Work out the finished part from the listing and answer in its coordinate system (mm). A direction names the side the tool comes from. Round coordinates to 2 decimals unless told otherwise and drop trailing zeros. Loops run counter-clockwise (first coordinate to the right, second up) from the corner with the lowest first, then second, coordinate; pieces in that order, holes last. Notation, with made-up numbers: (10, 24.5) -> (20, 24.5) arc R22 cw to (20, 34.5) -> close; hole circle Ø10 at (74.25, 57.25). An arc over 180 degrees is marked (long way). Write item = value, one per line. Start each with the question number.
Autodesk Inventor part; units mm, degrees
ref_plane "YZ Plane" through (0, 0, 0) normal (1, 0, 0) x (0, 1, 0)
ref_plane "XZ Plane" through (0, 0, 0) normal (0, 1, 0) x (-1, 0, 0)
ref_plane "XY Plane" through (0, 0, 0) normal (0, 0, 1) x (1, 0, 0)
sketch "Skizze3" plane through (0, 0, 0) normal (0, 0, 1) x (1, 0, 0)
  line L0 (0, 0) -> (-40, 0)
  line L1 (-40, 0) -> (-40, 35)
  line L2 (-40, 35) -> (0, 35)
  line L3 (0, 35) -> (0, 0)
  point P0 (-3.7, 3.7)
  dimension "d4" = 35
  dimension "d5" = 40
  dimension "d6" = 3.7
  dimension "d7" = 3.7
sketch "Skizze4" plane through (0, 0, 0) normal (0, 1, 0) x (-1, 0, 0)
  line L0 (0, 0) -> (40, 0)
  line L1 (20, 0) -> (20, 40)
  line L2 (20, 33) -> (20, 27) construction
  line L3 (26, 33) -> (26, 27)
  line L4 (14, 27) -> (14, 33)
  arc A0 (26, 33) -> (14, 33) centre (20, 33) ccw
  arc A1 (14, 27) -> (26, 27) centre (20, 27) ccw
  circle A2 centre (20, 30) radius 10
  line L5 (29.9773, 29.3273) -> (28, 0)
  line L6 (10.0227, 29.3273) -> (12, 0)
  dimension "d8" = 40
  dimension "d9" = 10
  dimension "d10" = 12
  dimension "d11" = 6
  dimension "d12" = 8
  dimension "d13" = 8
extrude "Extrusion3" add sketch "Skizze4" along normal blind 35 contours L6 A2 L1 L0 | L1 A2 L5 L0 | A2 L1 A0 L4 A1 | L1 A1 L3 A0 A2
extrude "Extrusion4" add sketch "Skizze3" against normal blind 2
hole "Bohrung1" at (-3.7, 3.7, 0) direction (0, 0, -1) diameter 2.459 depth 8.8 countersink diameter 7 countersink angle 90
sketch "Skizze5" plane through (0, 0, 0) normal (1, 0, 0) x (0, 0, -1)
  line L0 (-40, 0) -> (-40, 35)
  line L1 (-40, 9.25) -> (-5, 9.25)
  line L2 (-5, 9.25) -> (-5, 25.75)
  line L3 (-5, 25.75) -> (-40, 25.75)
  line L4 (-40, 25.75) -> (-40, 9.25)
  point P0 (0, 0)
  point P1 (-40, 17.5)
  dimension "d25" = 16.5
  dimension "d26" = 35
extrude "Extrusion5" cut sketch "Skizze5" against normal through all
pattern_linear "Rechteckige Anordnung1" count 2 spacing 32.6 along (-1, 0, 0) count 2 spacing 27.6 along (0, 1, 0) of "Bohrung1"
fillet "Rundung2" radius 2 2 edges at (-12, 17.5, 0) (-28, 17.5, 0)
equation "\"d13\" = d12"
equation "\"d14\" = d4"
equation "\"d31\" = d5 - 2 * d6"
equation "\"d34\" = d4 - 2 * d7"
properties part number "BT101_trajan20_21" material "Kunststoff, undurchsichtig Schwarz"
Item 1: A tool of negligible diameter and unlimited length cuts with its end or side. For faces 1 (the flat face through (-28.26, 17.26, 3.84)), 2 (the cylindrical face through (-20, 30, 39)), 3 (the flat face through (-5, 18, 0)), from which of +Z, -Z, +X, -X, +Y, -Y can it reach the whole face along a straight path? Write none if from no direction.
Item 2: Section A-A (x = -20) is taken. Determine the outline of the cut face in (y, z).
Item 3: Section C-C (y = 3.7) is taken. Determine the outline of the cut face in (x, z).
Item 4: Section B-B (z = 16.5) is taken. Determine the outline of the cut face in (x, y).
Item 5: Flat-ended cylindrical pins translate along their axes: pin 1 (6 mm diameter, centred on x = -25, y = 28.5, fed in from +Z); pin 2 (8 mm diameter, centred on y = 31.5, z = 12, fed in from -X); pin 3 (6.5 mm diameter, centred on y = 31.5, z = 30.5, fed in from -X); pin 4 (6 mm diameter, centred on x = -7, z = 32.5, fed in from -Y). Find the tip coordinate at first contact, or state that the pin passes through.
Item 6: The mould has two halves that part along Z. Classify faces 4 (the flat face through (-35, 18, 0)), 5 (the flat face through (-18, 0, 14)), 6 (the cylindrical face through (-28.663, 17.745, 0.651)), 7 (the flat face through (-11.74, 17.26, 3.84)): pulls with the +Z half, pulls with the -Z half, needs draft (parallel to the pull), parting line crosses it, or undercut.
Item 7: Section D-D (y = 12) is taken. Determine the outline of the cut face in (x, z), then the cut area to 3 significant figures.
Item 8: Find the intervals of material crossed by line 1 along Y through (x, z) = (-17, 11); line 2 along Z through (x, y) = (-8, 33.5); line 3 along X through (y, z) = (3, 30), in increasing order. Write a range as [from, to].
Worked answers:
q1.face_1 = -X, +Y, -Y
q1.face_2 = +Y, -Y
q1.face_3 = +Z, +X, +Y, -Y
q2.outline = (0, -2) -> (35, -2) -> (35, 21) -> (25.75, 21) -> (25.75, 5) -> (9.25, 5) -> (9.25, 21) -> (0, 21) -> close; (0, 39) -> (9.25, 39) -> (9.25, 40) -> (0, 40) -> close; (25.75, 39) -> (35, 39) -> (35, 40) -> (25.75, 40) -> close
q3.outline = (-40, -2) -> (-37.8, -2) -> (-39.8, 0) -> (-40, 0) -> close; (-34.8, -2) -> (-5.2, -2) -> (-7.2, 0) -> (-9.86, 0) arc R2 cw to (-11.86, 2.13) -> (-10.02, 29.33) arc R10 ccw (long way) to (-29.98, 29.33) -> (-28.14, 2.13) arc R2 cw to (-30.14, 0) -> (-32.8, 0) -> close; (-2.2, -2) -> (0, -2) -> (0, 0) -> (-0.2, 0) -> close; hole (-26, 27) arc R6 ccw to (-14, 27) -> (-14, 33) arc R6 ccw to (-26, 33) -> close
q4.outline = (-29.11, 0) -> (-10.89, 0) -> (-10.89, 9.25) -> (-29.11, 9.25) -> close; (-29.11, 25.75) -> (-10.89, 25.75) -> (-10.89, 35) -> (-29.11, 35) -> close
q5.pin_1 = 39.8
q5.pin_2 = -29.08
q5.pin_3 = -30
q5.pin_4 = through
q6.face_4 = pulls with the +Z half
q6.face_5 = needs draft
q6.face_6 = undercut
q6.face_7 = undercut
q7.outline = (-40, -2) -> (0, -2) -> (0, 0) -> (-9.86, 0) arc R2 cw to (-11.86, 2.13) -> (-11.66, 5) -> (-28.34, 5) -> (-28.14, 2.13) arc R2 cw to (-30.14, 0) -> (-40, 0) -> close
q7.area = 164 mm2
q8.line_1 = [0, 9.25], [25.75, 35]
q8.line_2 = [-2, 0]
q8.line_3 = [-30, -26], [-14, -10]
